from build123d import *

# Parameters (mm, degrees)
F1_DEPTH = 25.4
F2_R     = 39.1903568665
F3_DEPTH = 5.08


with BuildPart() as f1:
    # F0 (on Top) → F1 (new body)
    with BuildSketch(Plane.XY):
        with BuildLine():
            ThreePointArc((-21.971, 9.8715757037), (-21.2167040506, 11.1973157351), (-20.955, 12.7))
            ThreePointArc((-20.955, 12.7), (-21.2167040506, 14.2026842649), (-21.971, 15.5284242963))
            ThreePointArc((-21.971, 15.5284242963), (-22.987, 12.7), (-21.971, 9.8715757037))
        make_face()
        with BuildLine():
            ThreePointArc((-21.971, 15.5284242963), (-21.2167040506, 14.2026842649), (-20.955, 12.7))
            ThreePointArc((-20.955, 12.7), (-21.2167040506, 11.1973157351), (-21.971, 9.8715757037))
            ThreePointArc((-21.971, 9.8715757037), (-18.3824406922, 8.2578647221), (-14.9189074762, 10.1248833882))
            ThreePointArc((-14.9189074762, 10.1248833882), (-14.307459218, 11.3484492736), (-14.097, 12.7))
            ThreePointArc((-14.097, 12.7), (-17.0393157351, 16.8832959494), (-21.971, 15.5284242963))
        make_face()
        with BuildLine():
            ThreePointArc((-21.971, 9.8715757037), (-22.987, 12.7), (-21.971, 15.5284242963))
            ThreePointArc((-21.971, 15.5284242963), (-28.0696752968, 16.2539919541), (-29.0716406137, 10.1945898132))
            ThreePointArc((-29.0716406137, 10.1945898132), (-25.6019978851, 8.2595921522), (-21.971, 9.8715757037))
        make_face()
        with BuildLine():
            ThreePointArc((-14.9189074762, 10.1248833882), (-18.3824406922, 8.2578647221), (-21.971, 9.8715757037))
            ThreePointArc((-21.971, 9.8715757037), (-25.6019978851, 8.2595921522), (-29.0716406137, 10.1945898132))
            Line((-29.0716406137, 10.1945898132), (-22.1151784062, 0))
            Line((-22.1151784062, 0), (-14.9189074762, 10.1248833882))
        make_face()
    extrude(amount=F1_DEPTH)



with BuildPart() as f1b:
    # F0 (on Top) → F1, piece 2 (new body)
    with BuildSketch(Plane.XY):
        with BuildLine():
            ThreePointArc((3.4295447311, 9.8715757037), (7.0605426162, 8.2595921522), (10.5301853448, 10.1945898132))
            ThreePointArc((10.5301853448, 10.1945898132), (11.1058066449, 11.388973213), (11.3035447311, 12.7))
            ThreePointArc((11.3035447311, 12.7), (8.361228996, 16.8832959494), (3.4295447311, 15.5284242963))
            ThreePointArc((3.4295447311, 15.5284242963), (4.1838406805, 14.2026842649), (4.4455447311, 12.7))
            ThreePointArc((4.4455447311, 12.7), (4.1838406805, 11.1973157351), (3.4295447311, 9.8715757037))
        make_face()
        with BuildLine():
            Line((3.5737231374, 0), (10.5301853448, 10.1945898132))
            ThreePointArc((10.5301853448, 10.1945898132), (7.0605426162, 8.2595921522), (3.4295447311, 9.8715757037))
            ThreePointArc((3.4295447311, 9.8715757037), (-0.1590145767, 8.2578647221), (-3.6225477926, 10.1248833882))
            Line((-3.6225477926, 10.1248833882), (3.5737231374, 0))
        make_face()
        with BuildLine():
            ThreePointArc((-3.6225477926, 10.1248833882), (-0.1590145767, 8.2578647221), (3.4295447311, 9.8715757037))
            ThreePointArc((3.4295447311, 9.8715757037), (2.4135447311, 12.7), (3.4295447311, 15.5284242963))
            ThreePointArc((3.4295447311, 15.5284242963), (-2.702968088, 16.2283202004), (-3.6225477926, 10.1248833882))
        make_face()
        with BuildLine():
            ThreePointArc((3.4295447311, 15.5284242963), (2.4135447311, 12.7), (3.4295447311, 9.8715757037))
            ThreePointArc((3.4295447311, 9.8715757037), (4.1838406805, 11.1973157351), (4.4455447311, 12.7))
            ThreePointArc((4.4455447311, 12.7), (4.1838406805, 14.2026842649), (3.4295447311, 15.5284242963))
        make_face()
    extrude(amount=F1_DEPTH)


with BuildPart() as f1c:
    # F0 (on Top) → F1, piece 3 (new body)
    with BuildSketch(Plane.XY):
        with BuildLine():
            ThreePointArc((10.0777297444, -3.81), (-8.4868707531, -3.9956055876), (-27.0514712505, -3.81))
            ThreePointArc((-27.0514712506, -3.81), (-8.4868707531, -17.2068977255), (10.0777297444, -3.81))
        make_face()
    extrude(amount=F1_DEPTH)


with BuildPart() as f1_1:
    add(f1.part)

    add(f1b.part)  # F3 merges F1b

    add(f1c.part)  # F3 merges F1c
    # F2 (on Top) → F3 (join)
    with BuildSketch(Plane.XY):
        with Locations((-8.4868707531, 2.3543944123)):
            Circle(F2_R)
    extrude(amount=F3_DEPTH)


solid = f1_1.part
Verification items for the finished model (mm, model axes). A direction names the side the tool comes from. Give positions to 0.01 mm unless a question says otherwise; leave off trailing zeros. Order: outer loops, then holes, each group sorted by start corner. A loop starts at its lowest first (then second) coordinate and runs counter-clockwise, first axis right, second up. Notation, with made-up numbers: M 76.25,-17.5 L 128.25,-17.5 A23 cw 128.25,15.5 Z; hole C 3.5,9 d5. An arc over 180 degrees is marked long. Answer as a JSON object with one key per item and string values. Group by question number.
1) Cross-section at C-C (y = -10). Enter the section's corners in (x, z).
2) Cross-section at A-A (z = 22). Enter the section's corners in (x, y) (3 decimals), then the cut area to 3 significant figures.
3) Cross-section at D-D (x = -13). Enter the section's corners in (y, z).
4) Scan lines: line 1 along X through (y, z) = (13, 7.5); line 2 along Z through (x, y) = (7, 19.5); line 3 along Y through (x, z) = (7.5, 22.25). Record each from-to range of solid material in increasing order. Write a range as [from, to].
5) Access from +Z, -Z, +X, -X, +Y, -Y to the whole of each face (thin tool, end or side, straight path). Record for faces 1 (the face through (-18.57, 4.99, 15.1)), 2 (the face through (-9, -9, 25.4)), 3 (the face through (-25.642, 5.169, 15.098)), 4 (the face through (-8.829, -17.204, 15.098)), 5 (the face through (7.003, 5.026, 15.098)).
6) Cross-section at B-B (x = -25.4). Enter the section's corners in (y, z) (3 decimals), then the cut area to 3 significant figures.
7) Mould release check, pull along X, two halves, no side actions. Record for faces 6 (the face through (-17, -35.9, 2.5)), 7 (the face through (-9, 3, 0)), 8 (the face through (-2.627, 16.286, 15.098)), 9 (the face through (-8.227, -3.996, 15.098)): released by +X, released by -X, zero draft, split by the parting line, or undercut.
8) Depth check by flat-ended pin: pin 1 Ø1 at (x, z) = (-26, 20) entering from -Y; pin 2 Ø5 at (x, z) = (-20.5, 12) entering from -Y; pin 3 Ø1 at (x, z) = (2, 9.5) entering from -Y. Enter the tip coordinate at first touch or a pass-through.
Result sheet:
{
 "1": {"outline": "M -45.68,0 L 28.71,0 L 28.71,5.08 L 6.68,5.08 L 6.68,25.4 L -23.65,25.4 L -23.65,5.08 L -45.68,5.08 Z"},
 "2": {"outline": "M -29.072,10.195 L -22.115,0 L -14.919,10.125 A4.445 ccw -21.971,15.528 A4.445 ccw Z; M -27.051,-3.81 A19.561 ccw 10.078,-3.81 A928.525 cw Z; M -3.623,10.125 L 3.574,0 L 10.53,10.195 A4.445 ccw 3.43,15.528 A4.445 ccw Z", "area": "697 mm2"},
 "3": {"outline": "M -36.58,0 L 41.28,0 L 41.28,5.08 L -3.98,5.08 L -3.98,25.4 L -16.68,25.4 L -16.68,5.08 L -36.58,5.08 Z"},
 "4": {"line 1": "x = [-29.83, -14.11], [-4.43, 11.29]", "line 2": "z = [0, 5.08]", "line 3": "y = [-8.92, -3.86], [5.75, 17.1]"},
 "5": {"face 1": "+Z", "face 2": "+Z, +X, -X, +Y, -Y", "face 3": "+Z, -X", "face 4": "+Z, -Y", "face 5": "+Z, +X"},
 "6": {"outline": "M -32.999,0 L 37.707,0 L 37.707,5.08 L 17.145,5.08 L 17.145,25.4 L 4.814,25.4 L 4.814,5.08 L -3.842,5.08 L -3.842,25.4 L -7.474,25.4 L -7.474,5.08 L -32.999,5.08 Z", "area": "684 mm2"},
 "7": {"face 6": "split by the parting line", "face 7": "zero draft", "face 8": "undercut", "face 9": "undercut"},
 "8": {"pin 1": "stops at y = -7.3", "pin 2": "stops at y = -14.74", "pin 3": "stops at y = -14.47"}
}
